Can you work these out from the model? Positions are in its coordinate system, mm. A direction names the side the tool comes from. Coordinates: 2 decimals unless noted, no trailing zeros. Write each loop counter-clockwise with the first axis right and the second up, starting at its lowest first coordinate (ties: lowest second). Pieces come first, ordered by that corner, then holes. Notation, with made-up numbers: (-18.75, 84.25) - (20.25, 84.25) arc R28 ccw to (20.25, 107.25) - close; hole circle Ø10 at (32, -27). An arc over 180 degrees is marked (long way). Write each question's results on one line, items separated by ' | '. Start each with the question number.
```python
from build123d import *

# Parameters (mm, degrees)
F1_DEPTH  = 101.6
F3_R      = 3.429
F4_DEPTH  = 6.35
F2_R      = 3.429
F5_DEPTH  = 6.35
F6_R      = 26.035
F7_DEPTH  = 6.35
F8_R      = 1.3589
F9_DEPTH  = 127.001
F11_DEPTH = 127.001
F13_DEPTH = 114.3


with BuildPart() as f1:
    # F0 (on Front) → F1 (new body, symmetric)
    with BuildSketch(Plane.XZ):
        Polygon((-57.15, -38.1), (-57.15, 31.75), (57.15, 31.75), (57.15, -38.1), (63.5, -38.1), (63.5, 38.1), (-63.5, 38.1), (-63.5, -38.1), align=None)
    extrude(amount=F1_DEPTH, both=True)

    # F3 (on face) → F4 (cut)
    with BuildSketch(Plane(origin=(-63.5, 0, 0), x_dir=(0, -1, 0), z_dir=(-1, 0, 0))):
        with Locations((-76.2, -25.4)):
            Circle(F3_R)
        with Locations((-25.4, -25.4)):
            Circle(F3_R)
        with Locations((25.4, -25.4)):
            Circle(F3_R)
        with Locations((76.2, -25.4)):
            Circle(F3_R)
    extrude(amount=-F4_DEPTH, mode=Mode.SUBTRACT)

    # F2 (on face) → F5 (cut)
    with BuildSketch(Plane.YZ.offset(63.5)):
        with Locations((-76.2, -25.4)):
            Circle(F2_R)
        with Locations((-25.4, -25.4)):
            Circle(F2_R)
        with Locations((25.4, -25.4)):
            Circle(F2_R)
        with Locations((76.2, -25.4)):
            Circle(F2_R)
    extrude(amount=-F5_DEPTH, mode=Mode.SUBTRACT)

    # F6 (on face) → F7 (cut)
    with BuildSketch(Plane.XY.offset(38.1)):
        Circle(F6_R)
    extrude(amount=-F7_DEPTH, mode=Mode.SUBTRACT)

    # F8 (on face) → F9 (cut, through all)
    with BuildSketch(Plane.YZ.offset(63.5)):
        with Locations((19.05, -4.7498)):
            Circle(F8_R)
        with Locations((31.75, -4.7498)):
            Circle(F8_R)
    extrude(amount=-F9_DEPTH, mode=Mode.SUBTRACT)

    # F10 (on face) → F11 (cut, through all)
    with BuildSketch(Plane.YZ.offset(63.5)):
        Polygon((-63.5, 38.1), (-101.6, 38.1), (-101.6, 0), align=None)
        Polygon((63.5, 38.1), (101.6, 0), (101.6, 38.1), align=None)
    extrude(amount=-F11_DEPTH, mode=Mode.SUBTRACT)

    # F12 (on face) → F13 (join, through all)
    with BuildSketch(Plane.YZ.offset(-57.15)):
        Polygon((-69.85, 31.75), (-101.6, 0), (-101.6, -38.1), (-95.25, -38.1), (-95.25, -2.630256), (-60.869744, 31.75), align=None)
        Polygon((95.25, -2.630256), (95.25, -38.1), (101.6, -38.1), (101.6, 0), (69.85, 31.75), (60.869744, 31.75), align=None)
    extrude(amount=F13_DEPTH)


solid = f1.part
```
Q1. I'm going to push a flat-ended pin straight in: pin 1 Ø4 at (x, z) = (49.5, 3) entering from +Y. Where does the tip first touch, or does it pass through?
Q2. If we section it at A-A (x = 0): Please give me the cut outline in (y, z) (3 decimals), then the cut area to 3 significant figures.
Q3. I need wall thicknesses on line 1 along Y through (x, z) = (-62, -25); line 2 along X through (y, z) = (6.5, -2); line 3 along Y through (x, z) = (-24, -22). Which ranges of each line are inside material? Lowest first, please. Write a range as from..to.
Q4. If we section it at D-D (y = 24): Please give me the cut outline in (x, z), then the cut area to 3 significant figures.
Q5. If we section it at C-C (z = 28): Please give me the cut outline in (x, y), then the cut area to 3 significant figures.
Q6. Thinking about a two-plate mould opening in X: for faces 3 (the face through (63.5, -1, -1)), 4 (the face through (-57.15, -1, -4)), 5 (the face through (60.37, 24.66, -28.75)), which applies, pulls with the +X half, pulls with the -X half, needs draft (parallel to the pull), parting line crosses it, or undercut?
Q7. If we section it at B-B (y = -12.5): Please give me the cut outline in (x, z), then the cut area to 3 significant figures.
Q8. For faces 1 (the face through (-0.9, -82.3, 19.3)), 2 (the face through (-0.8, -78.3, 14.32)), which set-ups out of +Z, -Z, +X, -X, +Y, -Y let a thin tool reach every point of the face, with its end or its side?
Answer list:
1) pin 1: stops at y = 100.6
2) outline: (-101.6, -38.1) - (-95.25, -38.1) - (-95.25, -2.63) - (-60.87, 31.75) - (-26.035, 31.75) - (-26.035, 38.1) - (-63.5, 38.1) - (-101.6, 0) - close; (26.035, 31.75) - (60.87, 31.75) - (95.25, -2.63) - (95.25, -38.1) - (101.6, -38.1) - (101.6, 0) - (63.5, 38.1) - (26.035, 38.1) - close | area: 1,580 mm2
3) line 1: y = -101.6..-79.61, -72.79..-28.81, -21.99..21.99, 28.81..72.79, 79.61..101.6 | line 2: x = -63.5..-57.15, 57.15..63.5 | line 3: y = -101.6..-95.25, 95.25..101.6
4) outline: (-63.5, -38.1) - (-57.15, -38.1) - (-57.15, -28.53) - (-63.5, -28.53) - close; (-63.5, -22.27) - (-57.15, -22.27) - (-57.15, 31.75) - (-10.09, 31.75) - (-10.09, 38.1) - (-63.5, 38.1) - close; (10.09, 31.75) - (57.15, 31.75) - (57.15, -22.27) - (63.5, -22.27) - (63.5, 38.1) - (10.09, 38.1) - close; (57.15, -38.1) - (63.5, -38.1) - (63.5, -28.53) - (57.15, -28.53) - close | area: 1,490 mm2
5) outline: (-63.5, -73.6) - (63.5, -73.6) - (63.5, 73.6) - (-63.5, 73.6) - close; hole (-57.15, -64.62) - (57.15, -64.62) - (57.15, 64.62) - (-57.15, 64.62) - close | area: 3,920 mm2
6) face 3: pulls with the +X half | face 4: undercut | face 5: needs draft
7) outline: (-63.5, -38.1) - (-57.15, -38.1) - (-57.15, 31.75) - (-22.84, 31.75) - (-22.84, 38.1) - (-63.5, 38.1) - close; (22.84, 31.75) - (57.15, 31.75) - (57.15, -38.1) - (63.5, -38.1) - (63.5, 38.1) - (22.84, 38.1) - close | area: 1,400 mm2
8) face 1: +Z, +X, -X, -Y | face 2: -Z
